from build123d import *

# Parameters (mm, degrees)
F0_R     = 3.18
F1_DEPTH = 2.9
F3_DEPTH = 18.87


with BuildPart() as f1:
    # F0 (on Front) → F1 (new body)
    with BuildSketch(Plane.XZ):
        with BuildLine():
            Line((0, 0), (26.51, 0))
            Line((26.51, 0), (26.51, 9))
            Line((26.51, 9), (6.23, 9))
            Line((6.23, 9), (6.23, 18))
            Line((6.23, 18), (-11.764806, 29.434014))
            ThreePointArc((-11.764806, 29.434014), (-19.474339, 20.164339), (-7.461201, 19.140478))
            Line((-7.461201, 19.140478), (0, 14.399584))
            Line((0, 14.399584), (0, 0))
        make_face()
        with Locations((-13.200586, 22.78732)):
            Circle(F0_R, mode=Mode.SUBTRACT)
    extrude(amount=F1_DEPTH)

    # F2 (on face) → F3 (join)
    with BuildSketch(Plane.XZ.offset(2.9)):
        Polygon((26.51, 9), (6.23, 9), (0, 9), (0, 6.1), (26.51, 6.1), align=None)
    extrude(amount=-F3_DEPTH)

    # F5: F1 across plane


with BuildPart() as f1_1:
    add(f1.part)
    add(f1.part.mirror(Plane.XZ.offset(-15.97)))


solid = f1_1.part
Read the model definition and answer for the solid it produces. Units are mm, in the model's axes. A direction names the side the tool comes from. Coordinates: 2 decimals unless noted, no trailing zeros. Order: outer loops, then holes, each group sorted by start corner. A loop starts at its lowest first (then second) coordinate and runs counter-clockwise, first axis right, second up. Notation, with made-up numbers: (53.5, 56.25) -> (101.5, 56.25) arc R15 cw to (101.5, 70.25) -> close; hole circle Ø9 at (32, 89.25). An arc over 180 degrees is marked (long way). Answer as a JSON object with one key per item and string values.
1) Each of these flat-tipped pins is pushed along its axis until it touches: pin 1 (0.9 mm diameter, centred on y = -1.5, z = 15.5, fed in from +X); pin 2 (10 mm diameter, centred on x = 11, y = 1.5, fed in from -Z); pin 3 (8 mm diameter, centred on x = 10, y = 18.5, fed in from -Z); pin 4 (11.5 mm diameter, centred on y = 16.5, z = 4.5, fed in from -X). Where does it stop, or does it pass through?
Model answer:
{"pin 1": "stops at x = 6.23", "pin 2": "stops at z = 0", "pin 3": "stops at z = 6.1", "pin 4": "stops at x = 0"}
2) The mould has two halves that part along X. Classify faces 6 (the face through (-7.1, 0, 19.4)), 7 (the face through (-15.54, -1.43, 24.94)), 8 (the face through (26.51, 16.2, 6.4)): released by +X, released by -X, zero draft, split by the parting line, or undercut.
Model answer:
{"face 6": "zero draft", "face 7": "undercut", "face 8": "released by +X"}
3) A tool of negligible diameter and unlimited length cuts with its end or side. For faces 1 (the face through (-7.1, 31.94, 19.4)), 2 (the face through (13, 31.94, 3)), 3 (the face through (0, 16, 7)), 4 (the face through (6.23, -1, 13)), 5 (the face through (-3.78, 33.37, 16.8)), from which of +Z, -Z, +X, -X, +Y, -Y can it reach the whole face along a straight path? Write none if from no direction.
Model answer:
{"face 1": "+Z, +X, -X", "face 2": "-Z, +X, -X", "face 3": "-Z, -X, +Y, -Y", "face 4": "+Z, +X, +Y, -Y", "face 5": "-Z, +Y, -Y"}
4) A cutting plane is placed at C-C, the plane y = 32.5. Determine the outline of the cut face in (x, z).
Model answer:
{"outline": "(-11.76, 29.43) arc R6.8 ccw (long way) to (-7.46, 19.14) -> (0, 14.4) -> (0, 0) -> (26.51, 0) -> (26.51, 9) -> (6.23, 9) -> (6.23, 18) -> close; hole circle Ø6.36 at (-13.2, 22.79)"}
5) Consider line 1 along Y through (x, z) = (1, 19.5); line 2 along Z through (x, y) = (2, 15); line 3 along Z through (x, y) = (-3.5, -1). Determine where each line is inside the solid, lowest interval first. Write a range as from..to.
Model answer:
{"line 1": "y = -2.9..0, 31.94..34.84", "line 2": "z = 6.1..9", "line 3": "z = 16.62..24.18"}
6) A cutting plane is placed at D-D, the plane z = 24.5. Determine the outline of the cut face in (x, y).
Model answer:
{"outline": "(-19.78, -2.9) -> (-15.88, -2.9) -> (-15.88, 0) -> (-19.78, 0) -> close; (-19.78, 31.94) -> (-15.88, 31.94) -> (-15.88, 34.84) -> (-19.78, 34.84) -> close; (-10.52, -2.9) -> (-4, -2.9) -> (-4, 0) -> (-10.52, 0) -> close; (-10.52, 31.94) -> (-4, 31.94) -> (-4, 34.84) -> (-10.52, 34.84) -> close"}
7) A cutting plane is placed at B-B, the plane x = -13.5. Determine the outline of the cut face in (y, z).
Model answer:
{"outline": "(-2.9, 15.99) -> (0, 15.99) -> (0, 19.62) -> (-2.9, 19.62) -> close; (-2.9, 25.95) -> (0, 25.95) -> (0, 29.58) -> (-2.9, 29.58) -> close; (31.94, 15.99) -> (34.84, 15.99) -> (34.84, 19.62) -> (31.94, 19.62) -> close; (31.94, 25.95) -> (34.84, 25.95) -> (34.84, 29.58) -> (31.94, 29.58) -> close"}
8) A cutting plane is placed at A-A, the plane z = 10.75. Determine the outline of the cut face in (x, y).
Model answer:
{"outline": "(0, -2.9) -> (6.23, -2.9) -> (6.23, 0) -> (0, 0) -> close; (0, 31.94) -> (6.23, 31.94) -> (6.23, 34.84) -> (0, 34.84) -> close"}
